Could you check a few things on this model? Use its own coordinates, in mm. A direction names the side the tool comes from. Coordinates: 2 decimals unless noted, no trailing zeros. Loops run counter-clockwise (first coordinate to the right, second up) from the corner with the lowest first, then second, coordinate; pieces in that order, holes last.
from build123d import *

# Parameters (mm, degrees)
F1_DEPTH = 76.2
F3_R     = 4.5085
F4_DEPTH = 101.6
F2_R     = 4.5085
F5_DEPTH = 584.2


with BuildPart() as f1:
    # F0 (on Front) → F1 (new body)
    with BuildSketch(Plane.XZ):
        Polygon((-69.243231, 104.089492), (-120.043231, 104.089492), (-120.043231, -99.110508), (32.356769, -99.110508), (32.356769, -48.310508), (-69.243231, -48.310508), align=None)
    extrude(amount=F1_DEPTH)

    # F3 (on Top) → F4 (cut)
    with BuildSketch(Plane.XY):
        with Locations((-5.743231, -38.1)):
            Circle(F3_R)
    extrude(amount=-F4_DEPTH, mode=Mode.SUBTRACT)

    # F2 (on face) → F5 (cut)
    with BuildSketch(Plane.YZ.offset(-69.243231)):
        with Locations((-38.1, 65.989492)):
            Circle(F2_R)
    extrude(amount=-F5_DEPTH, mode=Mode.SUBTRACT)


solid = f1.part
(1) Imagine slicing it at B-B, the plane y = -50.5. Write out the boundary of the cut face in (x, z).
Answers:
outline: (-120.04, -99.11) - (32.36, -99.11) - (32.36, -48.31) - (-69.24, -48.31) - (-69.24, 104.09) - (-120.04, 104.09) - close
(2) Imagine slicing it at A-A, the plane y = -38.1. Write out the boundary of the cut face in (x, z).
Answers:
outline: (-120.04, -99.11) - (-10.25, -99.11) - (-10.25, -48.31) - (-69.24, -48.31) - (-69.24, 61.48) - (-120.04, 61.48) - close; (-120.04, 70.5) - (-69.24, 70.5) - (-69.24, 104.09) - (-120.04, 104.09) - close; (-1.23, -99.11) - (32.36, -99.11) - (32.36, -48.31) - (-1.23, -48.31) - close
(3) Imagine slicing it at D-D, the plane x = -47.5. Write out the boundary of the cut face in (y, z).
Answers:
outline: (-76.2, -99.11) - (0, -99.11) - (0, -48.31) - (-76.2, -48.31) - close
(4) We'd pull the mould along X, two halves only. Please class faces 1 (the face through (-69.243, -38, 27)), 2 (the face through (-1.44, -36.75, -73.35)), 3 (the face through (-94, -38, 104.089)), 4 (the face through (-120.043, -38, 4)): +X half, -X half, draft (parallel to the pull), parting line (faces both ways), or undercut.
Answers:
face 1: +X half
face 2: undercut
face 3: draft
face 4: -X half
(5) I need wall thicknesses on probe 1 along Z at (x, y) = (-44.5, -68); probe 2 along X at (y, z) = (-12, 49.5); probe 3 along X at (y, z) = (-38, -70). Which ranges of each line are inside material? Lowest first, please.
Answers:
probe 1: z = -99.11 to -48.31
probe 2: x = -120.04 to -69.24
probe 3: x = -120.04 to -10.25, -1.24 to 32.36
(6) For pin 1 (11.5 mm diameter, centred on y = -38.1, z = 65.99, fed in from +X); pin 2 (5 mm diameter, centred on x = -44, y = -60.5, fed in from +Z), each with a flat end and sliding along its axis, tell me the tip position at first contact or that it passes through.
Answers:
pin 1: stops at x = -69.24
pin 2: stops at z = -48.31
(7) Imagine slicing it at C-C, the plane z = 19.5. Write out the boundary of the cut face in (x, y), and give its area (3 significant figures).
Answers:
outline: (-120.04, -76.2) - (-69.24, -76.2) - (-69.24, 0) - (-120.04, 0) - close
area: 3,870 mm2
(8) Which directions (+Z, -Z, +X, -X, +Y, -Y) give clear straight access to the entire face, cutting with the end or side of a thin tool? Please do faces 5 (the face through (-18, -38, -48.311)), 6 (the face through (-79, 0, -19)).
Answers:
face 5: +Z, +X, +Y, -Y
face 6: +Z, -Z, +X, -X, +Y
